Could you check a few things on this model? Use its own coordinates, in mm. Face numbers are marked on the shaded views. Give positions to 0.01 mm unless a question says otherwise; leave off trailing zeros. Order: outer loops, then holes, each group sorted by start corner. A loop starts at its lowest first (then second) coordinate and runs counter-clockwise, first axis right, second up. Notation, with made-up numbers: (15.5, 34) -> (47.5, 34) arc R20 ccw to (47.5, 48) -> close; hole circle Ø10 at (13.25, 2.5). An arc over 180 degrees is marked (long way). One line per item, written item: value.
```python
from build123d import *

# Parameters (mm, degrees)
CROQUIS1_R              = 14
SALIENTE_EXTRUIR1_DEPTH = 3
CROQUIS2_R              = 11.075
SALIENTE_EXTRUIR2_DEPTH = 120
CROQUIS10_R             = 9
CORTAR_EXTRUIR1_DEPTH   = 125.583305463


with BuildPart() as part:
    # Croquis1 → Saliente-Extruir1 (new body)
    with BuildSketch(Plane(origin=(0, 0, 0), x_dir=(1, 0, 0), z_dir=(0, 1, 0))):
        with Locations(Location((0, 0, 0), (0, 0, 270))):
            Circle(CROQUIS1_R)
    extrude(amount=SALIENTE_EXTRUIR1_DEPTH)

    # Croquis2 → Saliente-Extruir2 (add)
    with BuildSketch(Plane(origin=(0, 3, 0), x_dir=(1, 0, 0), z_dir=(0, 1, 0))):
        with Locations(Location((0, 0, 0), (0, 0, 270))):
            Circle(CROQUIS2_R)
    extrude(amount=SALIENTE_EXTRUIR2_DEPTH)

    # Croquis4 → Revolución1 (revolve)
    with BuildSketch(Plane.XY, mode=Mode.PRIVATE) as revoluci_n1_sk:
        Polygon((14, 3), (11.075, 3), (11.075, 123), align=None)
    revolve(revoluci_n1_sk.sketch.rotate(Axis((0, 0, 0), (0, 1, 0)), 90), axis=Axis((0, 0, 0), (0, 1, 0)))

    # Croquis10 → Cortar-Extruir1 (cut, through all)
    with BuildSketch(Plane(origin=(0, 123, 0), x_dir=(1, 0, 0), z_dir=(0, 1, 0))):
        with Locations(Location((0, 0, 0), (0, 0, 270))):
            Circle(CROQUIS10_R)
    extrude(amount=-CORTAR_EXTRUIR1_DEPTH, mode=Mode.SUBTRACT)

    # Croquis11 → Revolución2 (revolve)
    with BuildSketch(Plane.XY, mode=Mode.PRIVATE) as revoluci_n2_sk:
        Polygon((9, 123), (9, 105), (8.182624783, 123), align=None)
    revolve(revoluci_n2_sk.sketch.rotate(Axis((0, 123, 0), (0, -1, 0)), 90), axis=Axis((0, 123, 0), (0, -1, 0)))


solid = part.part
```
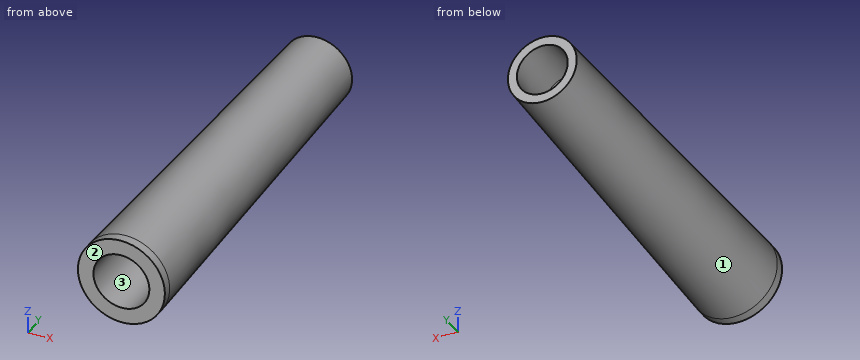
1) Suppose I cut it at A-A, the plane x = 0. Write out the boundary of the cut face in (y, z) (3 decimals).
Answer below:
outline: (0, -14) -> (3, -14) -> (123, -11.075) -> (123, -8.183) -> (105, -9) -> (0, -9) -> close; (0, 9) -> (105, 9) -> (123, 8.183) -> (123, 11.075) -> (3, 14) -> (0, 14) -> close
2) Suppose I cut it at D-D, the plane y = 54.5. Write out the boundary of the cut face in (x, z).
Answer below:
outline: circle Ø25.49 at (0, 0); hole circle Ø18 at (0, 0)
3) Suppose I cut it at C-C, the plane y = 99. Write out the boundary of the cut face in (x, z), then the cut area to 3 significant figures.
Answer below:
outline: circle Ø23.32 at (0, 0); hole circle Ø18 at (0, 0)
area: 173 mm2
4) We'd pull the mould along Z, two halves only. Please class the marked faces 1, 2 and 3: +Z half, -Z half, draft (parallel to the pull), parting line (faces both ways), or undercut.
Answer below:
face 1: parting line
face 2: draft
face 3: undercut
5) Suppose I cut it at B-B, the plane z = 0. Write out the boundary of the cut face in (x, y) (3 decimals), then the cut area to 3 significant figures.
Answer below:
outline: (-14, 0) -> (-9, 0) -> (-9, 105) -> (-8.183, 123) -> (-11.075, 123) -> (-14, 3) -> close; (8.183, 123) -> (9, 105) -> (9, 0) -> (14, 0) -> (14, 3) -> (11.075, 123) -> close
area: 894 mm2
6) If I drill on line 1 along Z through (x, y) = (0.75, 77); line 2 along X through (y, z) = (82.5, 8); line 3 along X through (y, z) = (24.5, -2), over which ranges is the centre line in solid material (lowest first)?
Answer below:
line 1: z = -12.17 to -8.97, 8.97 to 12.17
line 2: x = -9.03 to -4.12, 4.12 to 9.03
line 3: x = -13.33 to -8.77, 8.77 to 13.33
7) For P1, Ø2, axis at y = 69, z = 8, coming from the -X side; P2, Ø2, axis at x = -5.5, y = 49.5, coming from the -Z side; P3, Ø12, axis at x = 2, z = 8, coming from the -Y side; P4, Ø6, axis at x = 9.5, y = 88, coming from the +Z side, each with a flat end and sliding along its axis, tell me the tip position at first contact or that it passes through.
Answer below:
P1: stops at x = -10.23
P2: stops at z = -12.05
P3: stops at y = 0
P4: stops at z = 10
